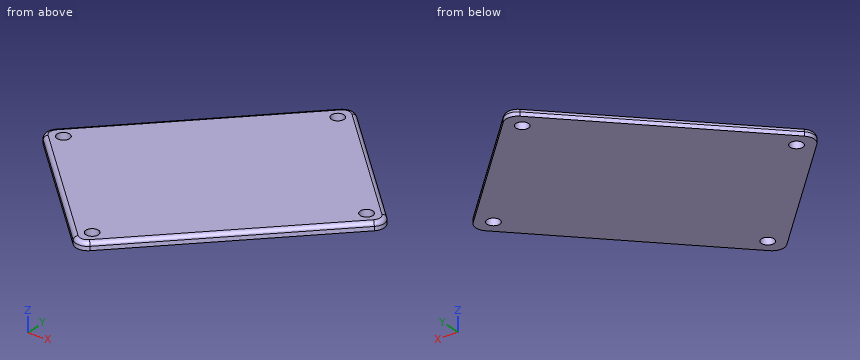
```python
from build123d import *

# Parameters (mm, degrees)
BOSS_EXTRUDE1_DEPTH = 2
CUT_EXTRUDE1_REACH  = 127.814
SKETCH2_R           = 1.6
FILLET1_R           = 1


with BuildPart() as part:
    # Sketch1 → Boss-Extrude1 (new body)
    with BuildSketch(Plane.XY):
        with BuildLine():
            Line((-75.603923459, -58.941906487), (-34.59173015, -17.929713178))
            ThreePointArc((-34.59173015, -17.929713178), (-33.713050494, -15.808392834), (-34.59173015, -13.687072491))
            Line((-34.59173015, -13.687072491), (-64.530631265, 16.251828625))
            ThreePointArc((-64.530631265, 16.251828625), (-66.651951609, 17.130508281), (-68.773271953, 16.251828625))
            Line((-68.773271953, 16.251828625), (-109.785465261, -24.760364684))
            ThreePointArc((-109.785465261, -24.760364684), (-110.664144918, -26.881685028), (-109.785465261, -29.003005371))
            Line((-109.785465261, -29.003005371), (-79.846564146, -58.941906487))
            ThreePointArc((-79.846564146, -58.941906487), (-77.725243802, -59.820586143), (-75.603923459, -58.941906487))
        make_face()
    extrude(amount=BOSS_EXTRUDE1_DEPTH)

    # Sketch2 → Cut-Extrude1 (cut, up to next)
    with BuildSketch(Plane.XY.offset(2), mode=Mode.PRIVATE) as cut_extrude1_sk1:
        with Locations((-106.329000575, -26.794058815)):
            Circle(SKETCH2_R)
    cut_extrude1_tool1 = extrude(cut_extrude1_sk1.sketch, amount=-CUT_EXTRUDE1_REACH, mode=Mode.PRIVATE) & part.part
    # Sketch2 → Cut-Extrude1 (cut, up to next)
    with BuildSketch(Plane.XY.offset(2), mode=Mode.PRIVATE) as cut_extrude1_sk2:
        with Locations(Location((-77.63761759, -55.4854418, 0), (0, 0, 180))):
            Circle(SKETCH2_R)
    cut_extrude1_tool2 = extrude(cut_extrude1_sk2.sketch, amount=-CUT_EXTRUDE1_REACH, mode=Mode.PRIVATE) & part.part
    # Sketch2 → Cut-Extrude1 (cut, up to next)
    with BuildSketch(Plane.XY.offset(2), mode=Mode.PRIVATE) as cut_extrude1_sk3:
        with Locations((-38.048194837, -15.896019047)):
            Circle(SKETCH2_R)
    cut_extrude1_tool3 = extrude(cut_extrude1_sk3.sketch, amount=-CUT_EXTRUDE1_REACH, mode=Mode.PRIVATE) & part.part
    # Sketch2 → Cut-Extrude1 (cut, up to next)
    with BuildSketch(Plane.XY.offset(2), mode=Mode.PRIVATE) as cut_extrude1_sk4:
        with Locations(Location((-66.739577822, 12.795363938, 0), (0, 0, 180))):
            Circle(SKETCH2_R)
    cut_extrude1_tool4 = extrude(cut_extrude1_sk4.sketch, amount=-CUT_EXTRUDE1_REACH, mode=Mode.PRIVATE) & part.part
    add(cut_extrude1_tool1.solids().sort_by_distance((-106.329001, -26.794059, 2))[0], mode=Mode.SUBTRACT)
    add(cut_extrude1_tool2.solids().sort_by_distance((-77.637618, -55.485442, 2))[0], mode=Mode.SUBTRACT)
    add(cut_extrude1_tool3.solids().sort_by_distance((-38.048195, -15.896019, 2))[0], mode=Mode.SUBTRACT)
    add(cut_extrude1_tool4.solids().sort_by_distance((-66.739578, 12.795364, 2))[0], mode=Mode.SUBTRACT)

    # Fillet1
    fillet1_edges = [part.edges().sort_by_distance(p)[0] for p in [
        (-77.725243802, -59.820586143, 2),
        (-55.097826804, -38.435809832, 2),
        (-33.713050494, -15.808392834, 2),
        (-49.561180708, 1.282378067, 2),
        (-66.651951609, 17.130508281, 2),
        (-89.279368607, -4.25426803, 2),
        (-110.664144918, -26.881685028, 2),
        (-94.816014704, -43.972455929, 2),
    ]]
    fillet(fillet1_edges, radius=FILLET1_R)


solid = part.part
```
Model file for the job. Use its own axes, mm. Coordinates: 2 decimals unless noted, no trailing zeros. Order: outer loops, then holes, each group sorted by start corner. A loop starts at its lowest first (then second) coordinate and runs counter-clockwise, first axis right, second up. Notation, with made-up numbers: (-31, -17.75) - (23, -17.75) arc R14 cw to (23, 6.25) - close; hole circle Ø5 at (73, 3.5). An arc over 180 degrees is marked (long way). Return JSON: item names as keys, results as strings. Group by question number.
1) Saw through at A-A, the plane z = 1.5. Write the cut outline in (x, y), plus the area to 3 significant figures.
2) Flat gauge pins, fed straight in: P1, Ø4, axis at x = -81.5, y = 3.5, coming from the +Z side; P2, Ø2.5, axis at x = -77.64, y = -55.49, coming from the -Z side. Where does each tip first touch, or does it go through?
3) Probe line 1 (Y direction, x = -107, z = 0.9); line 2 (X direction, y = -25.5, z = 1); line 3 (Y direction, x = -77.5, z = 1.2). List the from-to ranges inside material, lowest first. Write a range as from..to.
Values found:
{
 "1": {"outline": "(-109.69, -28.91) - (-79.75, -58.85) arc R2.87 ccw to (-75.7, -58.85) - (-34.69, -17.83) arc R2.87 ccw to (-34.69, -13.78) - (-64.63, 16.16) arc R2.87 ccw to (-68.68, 16.16) - (-109.69, -24.86) arc R2.87 ccw to start; hole circle Ø3.2 at (-106.33, -26.79); hole circle Ø3.2 at (-77.64, -55.49); hole circle Ø3.2 at (-66.74, 12.8); hole circle Ø3.2 at (-38.05, -15.9)", "area": "3,020 mm²"},
 "2": {"P1": "stops at z = 2", "P2": "passes through"},
 "3": {"line 1": "y = -31.79..-28.25, -25.34..-21.97", "line 2": "x = -110.33..-107.27, -105.39..-42.16", "line 3": "y = -59.79..-57.08, -53.89..7.5"}
}
